from build123d import *

# Parameters (mm, degrees)
BOSS_EXTRUDE1_DEPTH = 225
BOSS_EXTRUDE2_DEPTH = 5
BOSS_EXTRUDE3_DEPTH = 220
SKETCH4_W           = 140
SKETCH4_H           = 30
BOSS_EXTRUDE4_DEPTH = 5
BOSS_EXTRUDE5_DEPTH = 3
BOSS_EXTRUDE6_DEPTH = 3


with BuildPart() as part:
    # Sketch1 → Boss-Extrude1 (new body)
    with BuildSketch(Plane(origin=(0, 0, 0), x_dir=(1, 0, 0), z_dir=(0, 1, 0))):
        Polygon((0, 0), (0, 30), (3.4, 30), (3.4, 3.4), (30, 3.4), (30, 0), align=None)
    extrude(amount=BOSS_EXTRUDE1_DEPTH)

    # Sketch2 → Boss-Extrude2 (add)
    with BuildSketch(Plane(origin=(0, 0, 0), x_dir=(-1, 0, 0), z_dir=(0, -1, 0))):
        Polygon((-140, 0), (-30, 0), (-30, 3.4), (-3.4, 3.4), (-3.4, 30), (0, 30), (0, 30.423390593), (-140, 30.423390593), align=None)
    extrude(amount=-BOSS_EXTRUDE2_DEPTH)

    # Sketch3 → Boss-Extrude3 (add)
    with BuildSketch(Plane(origin=(0, 5, 0), x_dir=(1, 0, 0), z_dir=(0, 1, 0))):
        Polygon((140, 0), (140, 30.423390593), (136.6, 30.423390593), (136.6, 3.4), (110, 3.4), (110, 0), align=None)
    extrude(amount=BOSS_EXTRUDE3_DEPTH)

    # Sketch4 → Boss-Extrude4 (add)
    with BuildSketch(Plane(origin=(0, 225, 0), x_dir=(1, 0, 0), z_dir=(0, 1, 0))):
        with Locations((70, 15)):
            Rectangle(SKETCH4_W, SKETCH4_H)
    extrude(amount=BOSS_EXTRUDE4_DEPTH)

    # Sketch5 → Boss-Extrude5 (add)
    with BuildSketch(Plane(origin=(140, 0, 0), x_dir=(0, 0, -1), z_dir=(1, 0, 0))):
        Polygon((143.47826087, 30), (165, 0), (195, 0), (30, 230), (30, 225), (30.423390593, 225), (30.423390593, 187.591637355), align=None)
    extrude(amount=-BOSS_EXTRUDE5_DEPTH)

    # Sketch6 → Boss-Extrude6 (add)
    with BuildSketch(Plane.ZY):
        Polygon((-30, 230), (-195, 0), (-165, 0), (0, 230), align=None)
    extrude(amount=-BOSS_EXTRUDE6_DEPTH)


solid = part.part
Check sheet for the modelled part. Datum: model origin and axes. Units: mm. A direction names the side the tool comes from. Give positions to 0.01 mm unless a question says otherwise; leave off trailing zeros. Write each loop counter-clockwise with the first axis right and the second up, starting at its lowest first coordinate (ties: lowest second). Pieces come first, ordered by that corner, then holes. Notation, with made-up numbers: (86.25, 3) -> (123.25, 3) arc R11 cw to (123.25, 10) -> close; hole circle Ø10 at (74.5, 19.5). An arc over 180 degrees is marked (long way). Use one line per item in the form item = value. Start each with the question number.
1. Section check D-D (y = 162). Record the cut outline in (x, z).
2. Access from +Z, -Z, +X, -X, +Y, -Y to the whole of each face (thin tool, end or side, straight path). Record for faces 1 (the flat face through (3.4, 113, -17)), 2 (the flat face through (2, 167, -30)), 3 (the flat face through (3, 98, -107)), 4 (the flat face through (1.479, 116.61, -111.345)), 5 (the flat face through (22, 113, 0)).
3. Section check B-B (z = -162). Record the cut outline in (x, y).
4. Go/stop test with a flat-tipped pin: P1, Ø8, axis at x = 16, y = 117.5, coming from the -Z side. Record where the tip stops, or that it passes through.
5. Mould release check, pull along X, two halves, no side actions. Record for faces 6 (the flat face through (17, 113, -3.4)), 7 (the flat face through (71, 0, -15)), 8 (the flat face through (140, 124, -83)): pulls with the +X half, pulls with the -X half, needs draft (parallel to the pull), parting line crosses it, or undercut.
6. Section check C-C (x = 116). Record the cut outline in (y, z), and give its area (3 significant figures).
7. Section check A-A (x = 33). Record the cut outline in (y, z), and give its area (3 significant figures).
8. Thickness scan on line 1 along X through (y, z) = (24.5, -11); line 2 along X through (y, z) = (65, -122); line 3 along Z through (x, y) = (25, 177). Record the ranges inside material, lowest first. Write a range as from..to.
Conclusion:
q1.outline = (0, -78.78) -> (3, -78.78) -> (3, -48.78) -> (0, -48.78) -> close; (0, -30) -> (3.4, -30) -> (3.4, -3.4) -> (30, -3.4) -> (30, 0) -> (0, 0) -> close; (110, -3.4) -> (136.6, -3.4) -> (136.6, -30.42) -> (140, -30.42) -> (140, 0) -> (110, 0) -> close; (137, -78.78) -> (140, -78.78) -> (140, -48.78) -> (137, -48.78) -> close
q2.face_1 = -Z
q2.face_2 = none
q2.face_3 = -Z, +Y, -Y
q2.face_4 = -Z, +X, -X, +Y
q2.face_5 = +Z, +X, -X, +Y, -Y
q3.outline = (0, 4.18) -> (3, 4.18) -> (3, 46) -> (0, 46) -> close; (137, 4.18) -> (140, 4.18) -> (140, 46) -> (137, 46) -> close
q4.P1 = -3.4
q5.face_6 = undercut
q5.face_7 = needs draft
q5.face_8 = pulls with the +X half
q6.outline = (0, -30.42) -> (5, -30.42) -> (5, -3.4) -> (225, -3.4) -> (225, -30) -> (230, -30) -> (230, 0) -> (0, 0) -> close
q6.area = 1,050 mm²
q7.outline = (0, -30.42) -> (5, -30.42) -> (5, 0) -> (0, 0) -> close; (225, -30) -> (230, -30) -> (230, 0) -> (225, 0) -> close
q7.area = 302 mm²
q8.line_1 = 0..3.4, 136.6..140
q8.line_2 = 0..3, 137..140
q8.line_3 = -3.4..0
